```python
from build123d import *

# Parameters (mm, degrees)
CHAMFER2_SIZE                  = 8.144346428
CHAMFER2_SIZE_2                = 1
SKETCH8_R                      = 8.6
SKETCH8_R_2                    = 5.6
BOSS_EXTRUDE7_DEPTH            = 10
CUT_EXTRUDE1_REACH             = 35.014
CUT_EXTRUDE1_DIRECTION_2_REACH = 35.014
CHAMFER1_SIZE                  = 1
CHAMFER3_SIZE                  = 0.5
CHAMFER3_SIZE2                 = 0.288675135


with BuildPart() as part:
    # Sketch1 → Revolve1 (revolve)
    with BuildSketch(Plane.XY, mode=Mode.PRIVATE) as revolve1_sk:
        Polygon((-13.560768988, 5.5), (-17.5, 4.805407289), (-17.5, 0), (-12.05, 0), (-12.05, -0.35), (-11.05, -0.35), (-11.05, -10.35), (-5.6, -10.35), (-5.6, -10.1), (-3, -10.1), (-3, -16.35), (0, -16.35), (0, 5.5), align=None)
    revolve(revolve1_sk.sketch.rotate(Axis((0, -16.35, 0), (0, 1, 0)), 180), axis=Axis((0, -16.35, 0), (0, 1, 0)))

    # Chamfer2
    # the kernel refuses this chamfer: 8.144346428, 1 mm, written as the material it takes off along each edge
    with BuildSketch(Plane(origin=(0, 0, 0), x_dir=(1, 0, 0), z_dir=(0, 0, 1))) as chamfer2_piece_1_section:
        Polygon((17.5 - CHAMFER2_SIZE, 0), (17.5, CHAMFER2_SIZE_2), (17.5, 0), align=None)
    chamfer2_piece_1 = revolve(axis=Axis((0, 0, 0), (0, 1, 0)), mode=Mode.PRIVATE)
    chamfer2_piece_1 = chamfer2_piece_1 - Plane(origin=(0, 0.608985378, 0), x_dir=(1, 0, 0), z_dir=(0, -1, 0)) * Cylinder(12.05, 70, mode=Mode.PRIVATE)
    add(chamfer2_piece_1, mode=Mode.SUBTRACT)

    # Sketch8 → Boss-Extrude7 (add)
    with BuildSketch(Plane.XZ.offset(10.35)):
        Circle(SKETCH8_R)
        Circle(SKETCH8_R_2, mode=Mode.SUBTRACT)
    extrude(amount=BOSS_EXTRUDE7_DEPTH)

    # Cut-Extrude1: up to this face of the body (flat: up to its plane)
    cut_extrude1_end = Plane(part.part.faces().sort_by_distance((-5.441608081, -10.1, 0))[0])
    # Sketch2 → Cut-Extrude1 (cut, up to the picked face)
    with BuildSketch(Plane.XZ.offset(16.35), mode=Mode.PRIVATE) as cut_extrude1_sk1:
        Polygon((-6.25, 1.85), (-7, 1.1), (-7, -1.1), (-6.25, -1.85), (-0.75, -1.85), (0, -1.1), (0, 1.1), (-0.75, 1.85), align=None)
    cut_extrude1_tool1 = split(extrude(cut_extrude1_sk1.sketch, amount=-CUT_EXTRUDE1_REACH, mode=Mode.PRIVATE), bisect_by=cut_extrude1_end, keep=Keep.BOTH, mode=Mode.PRIVATE)
    add(cut_extrude1_tool1.solids().sort_by(Axis((-3.5, -16.35, 0), (0, 1, 0)))[0], mode=Mode.SUBTRACT)

    # Cut-Extrude1 direction 2: up to this face of the body (flat: up to its plane)
    cut_extrude1_direction_2_end = Plane(part.part.faces().sort_by_distance((-8.356755267, -20.35, 0))[0])
    # Sketch2 → Cut-Extrude1 direction 2 (cut, up to the picked face)
    with BuildSketch(Plane.XZ.offset(16.35), mode=Mode.PRIVATE) as cut_extrude1_direction_2_sk1:
        Polygon((-6.25, 1.85), (-7, 1.1), (-7, -1.1), (-6.25, -1.85), (-0.75, -1.85), (0, -1.1), (0, 1.1), (-0.75, 1.85), align=None)
    cut_extrude1_direction_2_tool1 = split(extrude(cut_extrude1_direction_2_sk1.sketch, amount=CUT_EXTRUDE1_DIRECTION_2_REACH, mode=Mode.PRIVATE), bisect_by=cut_extrude1_direction_2_end, keep=Keep.BOTH, mode=Mode.PRIVATE)
    add(cut_extrude1_direction_2_tool1.solids().sort_by(Axis((-3.5, -16.35, 0), (0, -1, 0)))[0], mode=Mode.SUBTRACT)

    # Chamfer1
    chamfer1_edges = [part.edges().sort_by_distance(p)[0] for p in [
        (5.6, -20.35, 0),
    ]]
    chamfer(chamfer1_edges, length=CHAMFER1_SIZE)

    # Chamfer3
    chamfer3_edges = [part.edges().sort_by_distance(p)[0] for p in [
        (-11.05, -10.35, 0),
    ]]
    chamfer3_side = [part.faces().sort_by_distance(p)[0] for p in [
        (-11.05, -5.35, 0),
    ]]
    chamfer(chamfer3_edges, length=CHAMFER3_SIZE, length2=CHAMFER3_SIZE2, reference=chamfer3_side[0])


solid = part.part
```
CAD build for the part. Positions are in the model's coordinates, mm. A direction names the side the tool comes from. Coordinates: 2 decimals unless noted, no trailing zeros. Order: outer loops, then holes, each group sorted by start corner. A loop starts at its lowest first (then second) coordinate and runs counter-clockwise, first axis right, second up. Notation, with made-up numbers: M 38.5,54.5 L 42.5,54.5 A17 ccw 42.5,85.5 Z; hole C -30,-9 d9. An arc over 180 degrees is marked long. Write each question's results on one line, items separated by ' | '. Start each with the question number.
Q1. Drill centre lines: probe 1 along Z at (x, y) = (2.5, -13); probe 2 along Z at (x, y) = (0, -16.5); probe 3 along Y at (x, z) = (-2, -11.5). Where is each one in solid material? Low to high. Write a range as from..to.
Q2. Cut at C-C (y = -6.75). List the corners of the cut face in (x, z), then the cut area to 3 significant figures.
Q3. Pull direction X, two halves, no side cores. Call faces 1 (the conical face through (5.755, -19.51, 0.232)), 2 (the flat face through (0, -13, 0)), 3 (the flat face through (11, -0.35, 4)), 4 (the cylindrical face through (-8.77, -5.17, 6.72)): +X half, -X half, draft (parallel to the pull), parting line (faces both ways), or undercut.
Q4. Flat gauge pins, fed straight in: P1, Ø3, axis at y = -2, z = 6.5, coming from the +X side; P2, Ø12, axis at y = -14.5, z = 1.5, coming from the -X side; P3, Ø1.8, axis at x = -1.5, y = -13.5, coming from the -Z side. Where does each tip first touch, or does it go through?
Q5. Cut at A-A (y = -14). List the corners of the cut face in (x, z).
Q6. Which spindle directions (+Z, -Z, +X, -X, +Y, -Y) get a long thin tool onto all of the face, cutting with end or side? Do faces 5 (the flat face through (0, 5.5, 0)), 6 (the cylindrical face through (-8.59, -15.28, 0.38)). Say none if no direction does.
Q7. Cut at D-D (y = 2.5). List the corners of the cut face in (x, z), then the cut area to 3 significant figures.
Found:
1) probe 1: -8.23..-5.01, -1.66..1.66, 5.01..8.23 | probe 2: -8.6..-5.6, 5.6..8.6 | probe 3: -0.35..5.5
2) outline: C 0,0 d22.1 | area: 384 mm²
3) face 1: undercut | face 2: undercut | face 3: draft | face 4: parting line
4) P1: x = 9.85 | P2: x = -11.05 | P3: z = -8.58
5) outline: C 0,0 d17.2; M -2.36,-1.85 A3 ccw long -2.36,1.85 L -0.75,1.85 L 0,1.1 L 0,-1.1 L -0.75,-1.85 Z; hole M -7,-1.1 L -6.25,-1.85 L -5.29,-1.85 A5.6 ccw long -5.29,1.85 L -6.25,1.85 L -7,1.1 Z
6) face 5: +Z, -Z, +X, -X, +Y | face 6: -Y
7) outline: C 0,0 d35 | area: 962 mm²
